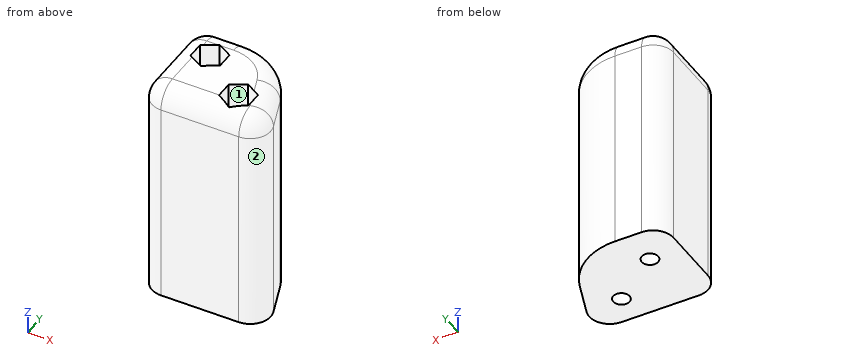
from build123d import *

# Parameters (mm, degrees)
PAD_DEPTH     = 55
FILLET_R      = 5
FILLET001_R   = 5
SKETCH004_R   = 2
HOLE001_DEPTH = 55.001
POCKET_START  = 30
POCKET_DEPTH  = 70


with BuildPart() as part:
    # Sketch → Pad (new body)
    with BuildSketch(Plane.XY):
        with BuildLine():
            Line((-10.503113, 0), (-22, 0))
            Line((-22, 0), (-22, -25))
            Line((-22, -25), (9.099256, -25))
            Line((3.592276, -9.869698), (9.099256, -25))
            ThreePointArc((3.592276, -9.869698), (-1.899467, -2.712719), (-10.503113, 0))
        make_face()
    extrude(amount=PAD_DEPTH)

    # Fillet
    fillet_edges = [part.edges().sort_by_distance(p)[0] for p in [
        (9.099256, -25, 27.5),
        (-22, -25, 27.5),
        (-22, 0, 27.5),
    ]]
    fillet(fillet_edges, radius=FILLET_R)

    # Fillet001
    fillet001_edges = [part.edges().sort_by_distance(p)[0] for p in [
        (-13.751557, 0, 55),
        (-20.535534, -1.464466, 55),
        (-1.899467, -2.712719, 55),
        (-22, -12.5, 55),
        (5.124628, -14.079799, 55),
        (-20.535534, -23.535534, 55),
        (6.054276, -22.867882, 55),
        (-7.520742, -25, 55),
    ]]
    fillet(fillet001_edges, radius=FILLET001_R)

    # Sketch004 → Hole001 (cut, through all)
    with BuildSketch(Plane.XY):
        with Locations((-2, -18)):
            Circle(SKETCH004_R)
        with Locations((-14, -9)):
            Circle(SKETCH004_R)
    extrude(amount=HOLE001_DEPTH, mode=Mode.SUBTRACT)

    # Sketch005 → Pocket (cut)
    with BuildSketch(Plane.XY.offset(POCKET_START)):
        Polygon((1.6, -15.921539), (-2, -13.843078), (-5.6, -15.921539), (-5.6, -20.078461), (-2, -22.156922), (1.6, -20.078461), align=None)
        Polygon((-10.4, -6.921539), (-14, -4.843078), (-17.6, -6.921539), (-17.6, -11.078461), (-14, -13.156922), (-10.4, -11.078461), align=None)
    extrude(amount=POCKET_DEPTH, mode=Mode.SUBTRACT)


solid = part.part
Build history of the part. All positions in model axes, mm. Face numbers are marked on the shaded views. A direction names the side the tool comes from. Coordinates: 2 decimals unless noted, no trailing zeros. Order: outer loops, then holes, each group sorted by start corner. A loop starts at its lowest first (then second) coordinate and runs counter-clockwise, first axis right, second up. Notation, with made-up numbers: M 67.5,32.5 L 85.5,32.5 A26 ccw 85.5,68.5 Z; hole C 7.5,-13.5 d2. An arc over 180 degrees is marked long. One line per question, with ' | ' between items. Start each with the question number.
Q1. 3-axis set-ups, long thin cutter, end or side, ignore diameter. For the marked faces 1 and 2: which of +Z, -Z, +X, -X, +Y, -Y reach the whole face in a straight line?
Q2. Probe L1, parallel to Y at x = -14, z = 15; L2, parallel to Z at x = -10, y = -20.5; L3, parallel to X at y = -10.25, z = 8. List the from-to ranges inside material, lowest first. Write a range as from..to.
Q3. Saw through at D-D (z = 52.5). List the corners of the cut face in (x, y), then the cut area to 3 significant figures.
Q4. Flat gauge pins, fed straight in: pin 1 Ø2 at (y, z) = (-6, 26) entering from +X; pin 2 Ø8 at (x, y) = (-11.5, -7) entering from +Z; pin 3 Ø4.5 at (y, z) = (-17, 42) entering from +X; pin 4 Ø10 at (x, y) = (2.5, -4) entering from +Z. Where does each tip first touch, or does it go through?
Q5. Saw through at A-A (z = 31). List the corners of the cut face in (x, y), then the cut area to 3 significant figures.
Q6. Saw through at B-B (y = -23.25). List the corners of the cut face in (x, z), then the cut area to 3 significant figures.
Q7. Saw through at C-C (z = 15.5). List the corners of the cut face in (x, y).
Check values:
1) face 1: +Z | face 2: +Z, -Z, +X
2) L1: y = -25..-11, -7..0 | L2: z = 0..54.97 | L3: x = -22..-15.56, -12.44..3.73
3) outline: M -21.33,-20 A4.33 ccw -17,-24.33 L 1.96,-24.33 A4.33 ccw 6.03,-18.52 L 2.96,-10.1 A14.33 ccw -10.5,-0.67 L -17,-0.67 A4.33 ccw -21.33,-5 Z; hole M -17.6,-11.08 L -14,-13.16 L -10.4,-11.08 L -10.4,-6.92 L -14,-4.84 L -17.6,-6.92 Z; hole M -5.6,-20.08 L -2,-22.16 L 1.6,-20.08 L 1.6,-15.92 L -2,-13.84 L -5.6,-15.92 Z | area: 470 mm2
4) pin 1: stops at x = 2.19 | pin 2: stops at z = 55 | pin 3: stops at x = 6.9 | pin 4: stops at z = 54.57
5) outline: M -22,-20 A5 ccw -17,-25 L 1.96,-25 A5 ccw 6.66,-18.29 L 3.59,-9.87 A15 ccw -10.5,0 L -17,0 A5 ccw -22,-5 Z; hole M -17.6,-11.08 L -14,-13.16 L -10.4,-11.08 L -10.4,-6.92 L -14,-4.84 L -17.6,-6.92 Z; hole M -5.6,-20.08 L -2,-22.16 L 1.6,-20.08 L 1.6,-15.92 L -2,-13.84 L -5.6,-15.92 Z | area: 531 mm2
6) outline: M -20.8,0 L 5.76,0 L 5.76,50 A3.8 ccw 1.96,53.8 L -17,53.8 A3.8 ccw -20.8,50 Z | area: 1,420 mm2
7) outline: M -22,-20 A5 ccw -17,-25 L 1.96,-25 A5 ccw 6.66,-18.29 L 3.59,-9.87 A15 ccw -10.5,0 L -17,0 A5 ccw -22,-5 Z; hole C -14,-9 d4; hole C -2,-18 d4
